Geometry check sheet. Reference: the model listing, model coordinates, mm. Coordinates: 2 decimals unless noted, no trailing zeros. Order: outer loops, then holes, each group sorted by start corner. A loop starts at its lowest first (then second) coordinate and runs counter-clockwise, first axis right, second up. Notation, with made-up numbers: (67, -23) - (71, -23) arc R22 cw to (71, -7) - close; hole circle Ø10 at (80.5, -8). An arc over 180 degrees is marked (long way). Put each result on its own line as item: value.
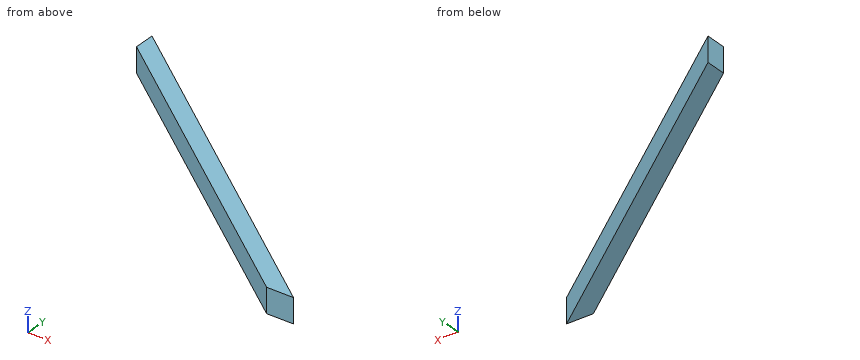
from build123d import *

# Parameters (mm, degrees)
BOSS_EXTRUDE1_DEPTH = 38.1
CUT_EXTRUDE1_DEPTH  = 127
CUT_EXTRUDE3_DEPTH  = 127


with BuildPart() as part:
    # Sketch1 → Boss-Extrude1 (new body)
    with BuildSketch(Plane.XY):
        Polygon((0, 398.78), (515.62, 0), (531.159215878, 20.092107154), (15.539215878, 418.872107154), align=None)
    extrude(amount=-BOSS_EXTRUDE1_DEPTH)

    # Sketch3 → Cut-Extrude1 (cut)
    with BuildSketch(Plane.XY):
        Polygon((15.539215878, 418.872107154), (15.539215878, 386.76198575), (0, 398.78), align=None)
    extrude(amount=-CUT_EXTRUDE1_DEPTH, mode=Mode.SUBTRACT)

    # Sketch4 → Cut-Extrude3 (cut)
    with BuildSketch(Plane.XY):
        Polygon((531.159215878, 20.092107154), (489.641033425, 20.092107154), (515.62, 0), align=None)
    extrude(amount=-CUT_EXTRUDE3_DEPTH, mode=Mode.SUBTRACT)


solid = part.part
Q1. Depth check by flat-ended pin: pin 1 Ø4 at (x, z) = (283.5, -15.5) entering from +Y; pin 2 Ø5 at (y, z) = (327.5, -20) entering from -X; pin 3 Ø6 at (y, z) = (62.5, -28.5) entering from +X. Enter the tip coordinate at first touch or a pass-through.
Answer block:
pin 1: stops at y = 213.18
pin 2: stops at x = 88.93
pin 3: stops at x = 480.21
Q2. Thickness scan on L1, parallel to Y at x = 222, z = -7; L2, parallel to X at y = 250.5, z = -19.5; L3, parallel to X at y = 340, z = -29. Record the ranges inside material, lowest first. Write a range as [from, to].
Answer block:
L1: y = [227.09, 259.2]
L2: x = [191.73, 233.24]
L3: x = [76, 117.52]
Q3. Section check A-A on z = -30. Record the boundary of the cut face in (x, y).
Answer block:
outline: (15.54, 386.76) - (489.64, 20.09) - (531.16, 20.09) - (15.54, 418.87) - close
Q4. Section check B-B on y = 84.5. Record the boundary of the cut face in (x, z), then the cut area to 3 significant figures.
Answer block:
outline: (406.36, -38.1) - (447.88, -38.1) - (447.88, 0) - (406.36, 0) - close
area: 1,580 mm^2
